```python
from build123d import *

# Parameters (mm, degrees)
SKETCH001_W     = 58
SKETCH001_H     = 45
PAD_DEPTH       = 14.15
SKETCH002_W     = 48
SKETCH002_H     = 35
POCKET_DEPTH    = 5
SKETCH004_R     = 2.5
POCKET001_DEPTH = 10
SKETCH_W        = 37
SKETCH_H        = 5
POCKET002_DEPTH = 5
SKETCH005_W     = 7.5
SKETCH005_H     = 5
POCKET003_DEPTH = 5


with BuildPart() as part:
    # Sketch001 → Pad (new body)
    with BuildSketch(Plane.XZ):
        with Locations((0, 17.5)):
            Rectangle(SKETCH001_W, SKETCH001_H)
    extrude(amount=PAD_DEPTH)

    # Sketch002 → Pocket (cut)
    with BuildSketch(Plane(origin=(0, 0, 0), x_dir=(1, 0, 0), z_dir=(0, 1, 0))):
        with Locations((0, -17.5)):
            Rectangle(SKETCH002_W, SKETCH002_H)
    extrude(amount=-POCKET_DEPTH, mode=Mode.SUBTRACT)

    # Sketch004 → Pocket001 (cut)
    with BuildSketch(Plane(origin=(0, -5, 0), x_dir=(1, 0, 0), z_dir=(0, 1, 0))):
        with Locations((-18.5, -9)):
            Circle(SKETCH004_R)
        with Locations((18.5, -9)):
            Circle(SKETCH004_R)
        with Locations((-18.5, -30)):
            Circle(SKETCH004_R)
        with Locations((18.5, -30)):
            Circle(SKETCH004_R)
    extrude(amount=-POCKET001_DEPTH, mode=Mode.SUBTRACT)

    # Sketch → Pocket002 (cut)
    with BuildSketch(Plane(origin=(0, 0, 40), x_dir=(-1, 0, 0), z_dir=(0, 0, 1))):
        with Locations((0, 2.5)):
            Rectangle(SKETCH_W, SKETCH_H)
    extrude(amount=-POCKET002_DEPTH, mode=Mode.SUBTRACT)

    # Sketch005 → Pocket003 (cut)
    with BuildSketch(Plane(origin=(0, 0, 0), x_dir=(-1, 0, 0), z_dir=(0, 0, 1))):
        with Locations((13.25, 2.5)):
            Rectangle(SKETCH005_W, SKETCH005_H)
        with Locations((-13.25, 2.5)):
            Rectangle(SKETCH005_W, SKETCH005_H)
    extrude(amount=-POCKET003_DEPTH, mode=Mode.SUBTRACT)


solid = part.part
```
Verification items for the finished model (mm, model axes). A direction names the side the tool comes from. Give positions to 0.01 mm unless a question says otherwise; leave off trailing zeros. Order: outer loops, then holes, each group sorted by start corner. A loop starts at its lowest first (then second) coordinate and runs counter-clockwise, first axis right, second up. Notation, with made-up numbers: M -9.75,36.5 L 42.25,36.5 A12 cw 42.25,53.5 Z; hole C 1.5,34.5 d10. An arc over 180 degrees is marked long. Answer in a Markdown table with one row per item. Add a question column.
Item 1: Section check A-A, the plane z = 9. Enter the section's corners in (x, y), and give its area (3 significant figures).
Item 2: Scan lines: probe 1 along Z at (x, y) = (-18.5, -9.75); probe 2 along X at (y, z) = (-10.25, 30); probe 3 along X at (y, z) = (-3, 27). Record each from-to range of solid material in increasing order. Write a range as from..to.
Item 3: Section check B-B, the plane y = -6.5. Enter the section's corners in (x, z), and give its area (3 significant figures).
Item 4: Gauge pin test, flat end, axial feed: pin 1 (12 mm diameter, centred on x = 14, z = 5.5, fed in from +Y). Record the tip position at first contact, or that the pin passes through.
Item 5: Mould release check, pull along Z, two halves, no side actions. Record for faces 1 (the flat face through (29, -7, 17)), 2 (the flat face through (0, -2, 0)), 3 (the flat face through (-24, -2, 18)): released by +Z, released by -Z, zero draft, split by the parting line, or undercut.
Item 6: Tool access check on faces 4 (the flat face through (21, -2, 35)), 5 (the flat face through (18.5, -2, 38)), 6 (the flat face through (9.5, -2, -2)). Record the directions out of +Z, -Z, +X, -X, +Y, -Y that give a thin tool (end or side, any length) a straight path to the whole face; none if there is none.
Item 7: Section check C-C, the plane z = -1. Enter the section's corners in (x, y), and give its area (3 significant figures).
Item 8: Section check D-D, the plane x = -0.5. Enter the section's corners in (y, z).
Filled sheet:
| question | item | result |
|---|---|---|
| 1 | outline | M -29,-14.15 L -21,-14.15 L -21,-5 L -24,-5 L -24,0 L -29,0 Z; M -16,-14.15 L 16,-14.15 L 16,-5 L -16,-5 Z; M 21,-14.15 L 29,-14.15 L 29,0 L 24,0 L 24,-5 L 21,-5 Z |
| 1 | area | 489 mm^2 |
| 2 | probe 1 | z = -5..6.5, 11.5..27.5, 32.5..40 |
| 2 | probe 2 | x = -29..-21, -16..16, 21..29 |
| 2 | probe 3 | x = -29..-24, 24..29 |
| 3 | outline | M -29,-5 L 29,-5 L 29,40 L -29,40 Z; hole C -18.5,9 d5; hole C -18.5,30 d5; hole C 18.5,9 d5; hole C 18.5,30 d5 |
| 3 | area | 2,530 mm^2 |
| 4 | pin 1 | stops at y = -5 |
| 5 | face 1 | zero draft |
| 5 | face 2 | released by +Z |
| 5 | face 3 | undercut |
| 6 | face 4 | +Y |
| 6 | face 5 | +Z, +Y |
| 6 | face 6 | +Z, -Z, +Y |
| 7 | outline | M -29,-14.15 L 29,-14.15 L 29,0 L 17,0 L 17,-5 L 9.5,-5 L 9.5,0 L -9.5,0 L -9.5,-5 L -17,-5 L -17,0 L -29,0 Z |
| 7 | area | 746 mm^2 |
| 8 | outline | M -14.15,-5 L 0,-5 L 0,0 L -5,0 L -5,40 L -14.15,40 Z |
